Autodesk Inventor part; units mm, degrees
ref_plane "YZ Plane" through (0, 0, 0) normal (1, 0, 0) x (0, 1, 0)
ref_plane "XZ Plane" through (0, 0, 0) normal (0, 1, 0) x (-1, 0, 0)
ref_plane "XY Plane" through (0, 0, 0) normal (0, 0, 1) x (1, 0, 0)
sketch "Sketch1" plane through (0, 0, 0) normal (0, 0, 1) x (1, 0, 0)
  circle A0 centre (-141.2963, -27.3767) radius 11
  line L0 (-141.2963, -11.3767) -> (-149.2963, -11.3767)
  line L1 (-152.2963, -14.3767) -> (-152.2963, -27.3767)
  line L2 (-152.2963, -27.3767) -> (-152.2963, -40.3767)
  line L3 (-141.2963, -11.3767) -> (-138.2963, -11.3767)
  line L4 (-138.2963, -11.3767) -> (-138.2963, -8.3767)
  line L5 (-138.2963, -8.3767) -> (-70.2823, -8.3767)
  line L6 (-141.2963, -46.3767) -> (-70.2823, -46.3767)
  line L7 (-141.2963, -46.3767) -> (-141.2963, -43.3767)
  line L8 (-141.2963, -43.3767) -> (-149.2963, -43.3767)
  arc A1 (-149.2963, -11.3767) -> (-152.2963, -14.3767) centre (-149.2963, -14.3767) ccw
  arc A2 (-152.2963, -40.3767) -> (-149.2963, -43.3767) centre (-149.2963, -40.3767) ccw
  line L9 (-23.7963, -41.3767) -> (-13.2963, -41.3767)
  line L10 (-13.2963, -41.3767) -> (10.1436, -38.2818)
  arc A3 (10.1436, -38.2818) -> (10.1436, -16.4717) centre (8.7037, -27.3767) ccw
  line L11 (10.1436, -16.4717) -> (-13.2963, -13.3767)
  line L12 (-13.2963, -13.3767) -> (-37.5536, -13.3767)
  circle A4 centre (8.7037, -27.3767) radius 4
  line L13 (-37.5536, -13.3767) -> (-37.5536, -8.3767)
  line L14 (-37.5536, -8.3767) -> (-70.2823, -8.3767)
  line L15 (-70.2823, -46.3767) -> (-37.5536, -46.3767)
  line L16 (-37.5536, -46.3767) -> (-37.5536, -41.3767)
  line L17 (-23.7963, -41.3767) -> (-37.5536, -41.3767)
  dimension "d18" = 22
  dimension "d20" = 16
  dimension "d22" = 3
  dimension "d27" = 3
extrude "Extrusion6" add sketch "Sketch1" along normal mid plane 111.5 contours A0 | L1 A1 L0 L3 L4 L5 L14 L13 L12 L11 A3 L10 L9 L17 L16 L15 L6 L7 L8 A2 L2
sketch "Sketch5" plane through (-138.2963, -8.3767, 55.75) normal (0, 1, 0) x (1, 0, 0)
  line L0 (100.7426, 0) -> (100.7426, 111.5)
  line L1 (100.7426, 0) -> (100.7426, 3)
  line L2 (100.7426, 3) -> (159.7547, 3)
  line L3 (100.7426, 111.5) -> (100.7426, 108.5)
  line L4 (100.7426, 108.5) -> (159.7547, 108.5)
  line L5 (159.7547, 108.5) -> (159.7547, 3)
  line L6 (100.7426, 3) -> (100.7426, 108.5)
  line L7 (157.9988, 3) -> (119.4988, 3)
  line L8 (119.4988, 3) -> (119.4988, 108.5)
  point P0 (138.2963, 55.75)
  dimension "d32" = 3
  dimension "d33" = 3
  dimension "d34" = 38.5
extrude "Extrusion7" cut sketch "Sketch5" against normal blind 105.5 contours L8 L4 L5 L2
sketch "Sketch6" plane through (-138.2963, -8.3767, 55.75) normal (0, 1, 0) x (1, 0, 0)
  line L0 (0, 0) -> (100.7426, 0)
  line L1 (100.7426, 111.5) -> (0, 111.5)
  line L2 (-11, 0) -> (0, 0)
  line L3 (0, 0) -> (0, 111.5)
  line L4 (0, 111.5) -> (-11, 111.5)
  line L5 (-11, 0) -> (-11, 111.5)
  line L6 (125, 3) -> (119.4988, 3)
  line L7 (119.4988, 3) -> (119.4988, 108.5)
  line L8 (119.4988, 108.5) -> (125, 108.5)
  line L9 (125, 108.5) -> (125, 111.5)
  line L10 (125, 111.5) -> (100.7426, 111.5)
  line L11 (100.7426, 0) -> (100.7426, 111.5)
  line L12 (100.7426, 0) -> (125, 0)
  line L13 (125, 0) -> (125, 3)
  line L14 (-14, 0) -> (-11, 0)
  line L15 (-11, 0) -> (-11, 111.5)
  line L16 (-11, 111.5) -> (-14, 111.5)
  line L17 (-14, 0) -> (-14, 111.5)
  line L18 (-14, 0) -> (-14, 111.5)
  line L19 (-14, 0) -> (-14, 111.5)
  line L20 (-14, 55.75) -> (-3, 55.75)
  line L21 (-3, 55.75) -> (-3, 74.75)
  line L22 (-3, 74.75) -> (-14, 74.75)
  line L23 (-3, 55.75) -> (-3, 36.75)
  line L24 (-3, 36.75) -> (-14, 36.75)
  line L25 (-11, 55.75) -> (42, 55.75)
  line L26 (42, 55.75) -> (42, 78.75)
  line L27 (42, 78.75) -> (74.75, 111.5)
  line L28 (-3, 74.75) -> (42, 74.75)
  line L29 (42, 55.75) -> (42, 32.75)
  line L30 (42, 32.75) -> (74.75, 0)
  line L31 (-3, 36.75) -> (42, 36.75)
  line L32 (74.75, 111.5) -> (-14, 111.5)
  line L33 (-14, 111.5) -> (-14, 74.75)
  line L34 (-14, 36.75) -> (-14, 0)
  line L35 (-14, 0) -> (74.75, 0)
  point P0 (138.2963, 55.75)
  dimension "d37" = 11
  dimension "d38" = 19
  dimension "d39" = 19
  dimension "d40" = 53
  dimension "d41" = 23
  dimension "d42" = 135
  dimension "d43" = 23
extrude "Extrusion8" cut sketch "Sketch6" against normal blind 105.5 contours L3 L31 L29 L30 L0 | L2 L5 L24 L31 L3 | L14 L17 L24 L5 | L28 L22 L5 L4 L3 | L3 L1 L27 L26 L28 | L22 L17 L16 L5
extrude "Extrusion9" add sketch "Sketch1" along normal mid plane 42 contours A0
properties part number "ForeArm"
Verification items for the finished model (mm, model axes). A direction names the side the tool comes from. Give positions to 0.01 mm unless a question says otherwise; leave off trailing zeros. Write each loop counter-clockwise with the first axis right and the second up, starting at its lowest first coordinate (ties: lowest second). Pieces come first, ordered by that corner, then holes. Notation, with made-up numbers: (-36.75, -1.5) -> (-16.75, -1.5) arc R20 cw to (-16.75, 21.5) -> close; hole circle Ø11 at (51.5, -12). An arc over 180 degrees is marked (long way). Use CSV: the item, a comma, the result in double quotes.
(1) Release check for a two-part mould opening along X. For faces 4 (the flat face through (-152.296, -27, 0)), 5 (the cylindrical face through (-152.286, -27.86, 19.986)), 6 (the flat face through (-144, -11.377, 0)) record: +X half, -X half, draft (parallel to the pull), parting line (faces both ways), or undercut.
Derived:
face 4,"-X half"
face 5,"undercut"
face 6,"draft"
(2) Set-up check for faces 1 (the flat face through (-118, -27, 19)), 2 (the flat face through (-28, -13.377, -1)), 3 (the flat face through (-145, -43.377, 0)): record each of +Z, -Z, +X, -X, +Y, -Y from which the full face is reachable in a straight line by a thin tool's end or side.
Derived:
face 1,"+Z"
face 2,"+Z, -Z, +X, +Y"
face 3,"+Z, -Z, -X, -Y"
(3) Material ranges on L1, parallel to Z at x = -1.5, y = -16; L2, parallel to X at y = -10, z = -14.5; L3, parallel to X at y = -43, z = 21, recorded low to high.
Derived:
L1,"z = -55.75 to -52.75, 52.75 to 55.75"
L2,"x = -138.3 to -37.55"
L3,"x = -96.3 to -37.55"
(4) Sectioned sample at C-C (x = -134.5). Record the cut outline in (y, z), plus the area to 3 significant figures.
Derived:
outline,"(-46.38, -19) -> (-36.03, -19) -> (-36.03, -21) -> (-18.73, -21) -> (-18.73, -19) -> (-8.38, -19) -> (-8.38, 19) -> (-18.73, 19) -> (-18.73, 21) -> (-36.03, 21) -> (-36.03, 19) -> (-46.38, 19) -> close"
area,"1,510 mm^2"
(5) Sectioned sample at D-D (z = -29). Record the cut outline in (x, y).
Derived:
outline,"(-90.3, -46.38) -> (-37.55, -46.38) -> (-37.55, -41.38) -> (-18.8, -41.38) -> (-18.8, -13.38) -> (-37.55, -13.38) -> (-37.55, -8.38) -> (-90.3, -8.38) -> close"
(6) Go/stop test with flat-tipped pins: pin 1 (1.5 mm diameter, centred on y = -44.5, z = 4.5, fed in from -X); pin 2 (2 mm diameter, centred on y = -24, z = -21, fed in from -X); pin 3 (3 mm diameter, centred on y = -29, z = 22, fed in from -X); pin 4 (6.5 mm diameter, centred on x = 8.7, y = -27.38, fed in from +Z). Record where each tip stops, or that it passes through.
Derived:
pin 1,"stops at x = -141.3"
pin 2,"stops at x = -152.04"
pin 3,"stops at x = -152.28"
pin 4,"passes through"
(7) Sectioned sample at A-A (z = -11). Record the cut outline in (x, y), plus the area to 3 significant figures.
Derived:
outline,"(-152.3, -40.38) arc R3 ccw to (-149.3, -43.38) -> (-141.3, -43.38) -> (-141.3, -46.38) -> (-37.55, -46.38) -> (-37.55, -41.38) -> (-18.8, -41.38) -> (-18.8, -13.38) -> (-37.55, -13.38) -> (-37.55, -8.38) -> (-138.3, -8.38) -> (-138.3, -11.38) -> (-149.3, -11.38) arc R3 ccw to (-152.3, -14.38) -> close"
area,"4,810 mm^2"
(8) Sectioned sample at B-B (y = -20.5). Record the cut outline in (x, z).
Derived:
outline,"(-152.3, -19) -> (-149.88, -19) -> (-149.88, -21) -> (-132.71, -21) -> (-132.71, -19) -> (-96.3, -19) -> (-96.3, -23) -> (-63.55, -55.75) -> (17.29, -55.75) -> (17.29, -52.75) -> (-18.8, -52.75) -> (-18.8, 52.75) -> (17.29, 52.75) -> (17.29, 55.75) -> (-63.55, 55.75) -> (-96.3, 23) -> (-96.3, 19) -> (-132.71, 19) -> (-132.71, 21) -> (-149.88, 21) -> (-149.88, 19) -> (-152.3, 19) -> close"
